Check sheet for the modelled part. Datum: model origin and axes. Units: mm. Give positions to 0.01 mm unless a question says otherwise; leave off trailing zeros. Order: outer loops, then holes, each group sorted by start corner. A loop starts at its lowest first (then second) coordinate and runs counter-clockwise, first axis right, second up.
from build123d import *

# Parameters (mm, degrees)
SKETCH1_W           = 110
SKETCH1_H           = 140
SKETCH1_R           = 2
BOSS_EXTRUDE1_DEPTH = 3.175
SKETCH3_R           = 45
SKETCH3_R_2         = 2
SKETCH3_R_3         = 13.5
SKETCH3_R_4         = 1.4732
BOSS_EXTRUDE3_DEPTH = 3.175
SKETCH4_W           = 110
SKETCH4_H           = 10
BOSS_EXTRUDE5_DEPTH = 3.175
FILLET1_R           = 6
SKETCH6_R           = 2
SKETCH6_R_2         = 13.5
CUT_EXTRUDE1_DEPTH  = 10


with BuildPart() as part:
    # Sketch1 → Boss-Extrude1 (new body)
    with BuildSketch(Plane.XY):
        Rectangle(SKETCH1_W, SKETCH1_H)
        with Locations((-47.5, 40)):
            Circle(SKETCH1_R, mode=Mode.SUBTRACT)
        with Locations((47.5, 40)):
            Circle(SKETCH1_R, mode=Mode.SUBTRACT)
        with Locations((-47.5, 60)):
            Circle(SKETCH1_R, mode=Mode.SUBTRACT)
        with Locations((47.5, 60)):
            Circle(SKETCH1_R, mode=Mode.SUBTRACT)
    extrude(amount=BOSS_EXTRUDE1_DEPTH)

    # Sketch3 → Boss-Extrude3 (add)
    # profile 1 of 2: a face of its own
    with BuildSketch(Plane.XY.offset(3.175)):
        with Locations((-50, -18)):
            Circle(SKETCH3_R)
        with Locations((-67.5, -18)):
            Circle(SKETCH3_R_2, mode=Mode.SUBTRACT)
        with Locations((-50, -18)):
            Circle(SKETCH3_R_3, mode=Mode.SUBTRACT)
        with Locations((-85.238473279, -5.174244625)):
            Circle(SKETCH3_R_4, mode=Mode.SUBTRACT)
    # profile 2 of 2: a face of its own
    with BuildSketch(Plane.XY.offset(3.175)):
        with Locations((50, -18)):
            Circle(SKETCH3_R)
        with Locations((67.5, -18)):
            Circle(SKETCH3_R_2, mode=Mode.SUBTRACT)
        with Locations((50, -18)):
            Circle(SKETCH3_R_3, mode=Mode.SUBTRACT)
        with Locations((85.238473279, -5.174244625)):
            Circle(SKETCH3_R_4, mode=Mode.SUBTRACT)
    extrude(amount=-BOSS_EXTRUDE3_DEPTH)

    # Sketch4 → Boss-Extrude5 (add)
    # profile 1 of 4: a face of its own
    with BuildSketch(Plane.XY.offset(3.175)):
        with BuildLine():
            ThreePointArc((-60, -61.874821937), (-63.111300905, -61.047575873), (-66.155494421, -60))
            Line((-66.155494421, -60), (-110, -60))
            Line((-110, -60), (-110, -130))
            Line((-110, -130), (-60, -130))
            Line((-60, -130), (-60, -121.715728753))
            Line((-60, -121.715728753), (-60, -61.874821937))
        make_face()
        with BuildLine():
            Line((-102.5, -122.95), (-97.5, -122.95))
            ThreePointArc((-97.5, -122.95), (-95.45, -125), (-97.5, -127.05))
            Line((-97.5, -127.05), (-102.5, -127.05))
            ThreePointArc((-102.5, -127.05), (-104.55, -125), (-102.5, -122.95))
        make_face(mode=Mode.SUBTRACT)
        with BuildLine():
            ThreePointArc((-97.5, -62.95), (-95.45, -65), (-97.5, -67.05))
            Line((-97.5, -67.05), (-102.5, -67.05))
            ThreePointArc((-102.5, -67.05), (-104.55, -65), (-102.5, -62.95))
            Line((-102.5, -62.95), (-97.5, -62.95))
        make_face(mode=Mode.SUBTRACT)
    # profile 2 of 4: a face of its own
    with BuildSketch(Plane.XY.offset(3.175)):
        with BuildLine():
            Line((-110, -60), (-66.155494421, -60))
            ThreePointArc((-66.155494421, -60), (-90.46935182, -37.678200204), (-93.011169428, -4.76975796))
            Line((-93.011169428, -4.76975796), (-110, -60))
        make_face()
    # profile 3 of 4: a face of its own
    with BuildSketch(Plane.XY.offset(3.175)):
        with BuildLine():
            ThreePointArc((-55, -62.72135955), (-57.51193427, -62.368579462), (-60, -61.874821937))
            Line((-60, -61.874821937), (-60, -121.715728753))
            Line((-60, -121.715728753), (-60, -130))
            Line((-60, -130), (0, -130))
            Line((0, -130), (0, -70))
            Line((0, -70), (-55, -70))
            Line((-55, -70), (-55, -62.72135955))
        make_face()
    # profile 4 of 4: a face of its own
    with BuildSketch(Plane.XY.offset(3.175)):
        with Locations((-55, -135)):
            Rectangle(SKETCH4_W, SKETCH4_H)
    boss_extrude5 = extrude(amount=-BOSS_EXTRUDE5_DEPTH)

    # Mirror2: Boss-Extrude5 across plane
    add(boss_extrude5.mirror(Plane(origin=(0, 0, 0), x_dir=(0, 0, 1), z_dir=(1, 0, 0))))

    # Fillet1
    fillet1_edges = [part.edges().sort_by_distance(p)[0] for p in [
        (-55, 26.72135955, 1.5875),
        (55, 26.72135955, 1.5875),
    ]]
    fillet(fillet1_edges, radius=FILLET1_R)

    # Sketch6 → Cut-Extrude1 (cut)
    with BuildSketch(Plane.XY.offset(3.175)):
        with Locations((32.5, -18)):
            Circle(SKETCH6_R)
        with Locations((50, -0.5)):
            Circle(SKETCH6_R)
        with Locations((67.5, -18)):
            Circle(SKETCH6_R)
        with Locations((50, -18)):
            Circle(SKETCH6_R_2)
        with Locations((50, -35.5)):
            Circle(SKETCH6_R)
        with Locations((-50, -18)):
            Circle(SKETCH6_R_2)
        with Locations((-67.5, -18)):
            Circle(SKETCH6_R)
        with Locations((-50, -35.5)):
            Circle(SKETCH6_R)
        with Locations((-32.5, -18)):
            Circle(SKETCH6_R)
        with Locations((-50, -0.5)):
            Circle(SKETCH6_R)
    extrude(amount=-CUT_EXTRUDE1_DEPTH, mode=Mode.SUBTRACT)


solid = part.part
1) Section check A-A, the plane y = -12.5. Record the cut outline in (x, z) (3 decimals).
Recorded:
outline: (-95.389, 0) - (-62.329, 0) - (-62.329, 3.175) - (-95.389, 3.175) - close; (-37.671, 0) - (37.671, 0) - (37.671, 3.175) - (-37.671, 3.175) - close; (62.329, 0) - (95.389, 0) - (95.389, 3.175) - (62.329, 3.175) - close
2) Section check C-C, the plane x = 78. Record the cut outline in (y, z) (3 decimals), then the cut area to 3 significant figures.
Recorded:
outline: (-140, 0) - (17.228, 0) - (17.228, 3.175) - (-140, 3.175) - close
area: 499 mm2
3) Section check B-B, the plane z = 0.65. State how many separate pieces and enclosed holes the cut face has, then the cut area to 3 significant figures.
Recorded:
separate pieces: 1
enclosed holes: 20
area: 37,300 mm2
4) Section check D-D, the plane x = -81. Record the cut outline in (y, z) (3 decimals), then the cut area to 3 significant figures.
Recorded:
outline: (-140, 0) - (14.619, 0) - (14.619, 3.175) - (-140, 3.175) - close
area: 491 mm2
5) Depth check by flat-ended pin: pin 1 Ø2.5 at (x, y) = (-32.5, -18) entering from +Z; pin 2 Ø6 at (x, y) = (45.5, 3.5) entering from -Z. Enter the tip coordinate at first touch or a pass-through.
Recorded:
pin 1: passes through
pin 2: stops at z = 0
6) Material ranges on L1, parallel to Y at x = -50, z = 1.8; L2, parallel to Y at x = 32.5, z = 1.2; L3, parallel to Y at x = -47.5, z = 1.75, recorded low to high.
Recorded:
L1: y = -140 to -37.5, -33.5 to -31.5, -4.5 to -2.5, 1.5 to 70
L2: y = -140 to -20, -16 to 70
L3: y = -140 to -31.27, -4.73 to 38, 42 to 58, 62 to 70
7) Draft check along X on faces 1 (the face through (2, -57, 0)), 2 (the face through (59.42, -8.33, 1.61)), 3 (the face through (101.387, -31.998, 1.61)). Enter one of: +X half, -X half, draft (parallel to the pull), parting line (faces both ways), or undercut.
Recorded:
face 1: draft
face 2: undercut
face 3: +X half
